CAD build for the part. Positions are in the model's coordinates, mm. Face numbers are marked on the shaded views. Round coordinates to 2 decimals unless told otherwise and drop trailing zeros. Loops run counter-clockwise (first coordinate to the right, second up) from the corner with the lowest first, then second, coordinate; pieces in that order, holes last. Notation, with made-up numbers: (-7, 54.25) - (30, 54.25) arc R28 cw to (30, 78.25) - close; hole circle Ø1 at (78, -1.75). An arc over 180 degrees is marked (long way). Use one line per item in the form item = value.
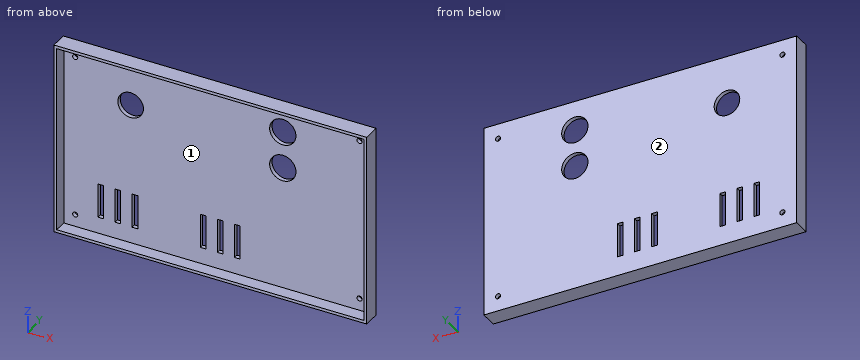
from build123d import *

# Parameters (mm, degrees)
SKETCH_1_W                       = 220
SKETCH_1_H                       = 135
LID_TOP_3MM_DEPTH                = 3
SKETCH_2_W                       = 216
SKETCH_2_H                       = 2
LID_RIM_BACK_DEPTH               = 12
SKETCH_3_W                       = 216
SKETCH_3_H                       = 2
LID_RIM_FRONT_DEPTH              = 12
SKETCH_4_W                       = 2
SKETCH_4_H                       = 135
LID_RIM_LEFT_DEPTH               = 12
SKETCH_5_W                       = 2
SKETCH_5_H                       = 135
LID_RIM_RIGHT_DEPTH              = 12
SKETCH_6_R                       = 1.8
LID_SCREW_CLEARANCE_1_DEPTH      = 16
SKETCH_7_R                       = 1.8
LID_SCREW_CLEARANCE_2_DEPTH      = 16
SKETCH_8_R                       = 1.8
LID_SCREW_CLEARANCE_3_DEPTH      = 16
SKETCH_9_R                       = 1.8
LID_SCREW_CLEARANCE_4_DEPTH      = 16
SKETCH_10_R                      = 9
OV5647_LENS_OPENING_D18_DEPTH    = 4
SKETCH_11_R                      = 9.25
HC_SR04_ACOUSTIC_OPENING_1_DEPTH = 4
SKETCH_12_R                      = 9.25
HC_SR04_ACOUSTIC_OPENING_2_DEPTH = 4
SKETCH_13_W                      = 4
SKETCH_13_H                      = 24
VENT_SLOT_1_DEPTH                = 4
SKETCH_14_W                      = 4
SKETCH_14_H                      = 24
VENT_SLOT_2_DEPTH                = 4
SKETCH_15_W                      = 4
SKETCH_15_H                      = 24
VENT_SLOT_3_DEPTH                = 4
SKETCH_16_W                      = 4
SKETCH_16_H                      = 24
VENT_SLOT_4_DEPTH                = 4
SKETCH_17_W                      = 4
SKETCH_17_H                      = 24
VENT_SLOT_5_DEPTH                = 4
SKETCH_18_W                      = 4
SKETCH_18_H                      = 24
VENT_SLOT_6_DEPTH                = 4


with BuildPart() as part:
    # 草图1 → Lid_Top_3mm (new body)
    with BuildSketch(Plane(origin=(0, 0, 0), x_dir=(1, 0, 0), z_dir=(0, 1, 0))):
        Rectangle(SKETCH_1_W, SKETCH_1_H)
    extrude(amount=-LID_TOP_3MM_DEPTH)

    # 草图2 → Lid_Rim_Back (add)
    with BuildSketch(Plane(origin=(0, 0, 0), x_dir=(1, 0, 0), z_dir=(0, 1, 0))):
        with Locations((0, 66.5)):
            Rectangle(SKETCH_2_W, SKETCH_2_H)
    extrude(amount=-LID_RIM_BACK_DEPTH)

    # 草图3 → Lid_Rim_Front (add)
    with BuildSketch(Plane(origin=(0, 0, 0), x_dir=(1, 0, 0), z_dir=(0, 1, 0))):
        with Locations((0, -66.5)):
            Rectangle(SKETCH_3_W, SKETCH_3_H)
    extrude(amount=-LID_RIM_FRONT_DEPTH)

    # 草图4 → Lid_Rim_Left (add)
    with BuildSketch(Plane(origin=(0, 0, 0), x_dir=(1, 0, 0), z_dir=(0, 1, 0))):
        with Locations((-109, 0)):
            Rectangle(SKETCH_4_W, SKETCH_4_H)
    extrude(amount=-LID_RIM_LEFT_DEPTH)

    # 草图5 → Lid_Rim_Right (add)
    with BuildSketch(Plane(origin=(0, 0, 0), x_dir=(1, 0, 0), z_dir=(0, 1, 0))):
        with Locations((109, 0)):
            Rectangle(SKETCH_5_W, SKETCH_5_H)
    extrude(amount=-LID_RIM_RIGHT_DEPTH)

    # 草图6 → Lid_Screw_Clearance_1 (cut)
    with BuildSketch(Plane(origin=(0, 0, 0), x_dir=(1, 0, 0), z_dir=(0, 1, 0))):
        with Locations(Location((-100, -57, 0), (0, 0, 270))):
            Circle(SKETCH_6_R)
    extrude(amount=-LID_SCREW_CLEARANCE_1_DEPTH, mode=Mode.SUBTRACT)

    # 草图7 → Lid_Screw_Clearance_2 (cut)
    with BuildSketch(Plane(origin=(0, 0, 0), x_dir=(1, 0, 0), z_dir=(0, 1, 0))):
        with Locations(Location((100, -57, 0), (0, 0, 270))):
            Circle(SKETCH_7_R)
    extrude(amount=-LID_SCREW_CLEARANCE_2_DEPTH, mode=Mode.SUBTRACT)

    # 草图8 → Lid_Screw_Clearance_3 (cut)
    with BuildSketch(Plane(origin=(0, 0, 0), x_dir=(1, 0, 0), z_dir=(0, 1, 0))):
        with Locations(Location((-100, 57, 0), (0, 0, 270))):
            Circle(SKETCH_8_R)
    extrude(amount=-LID_SCREW_CLEARANCE_3_DEPTH, mode=Mode.SUBTRACT)

    # 草图9 → Lid_Screw_Clearance_4 (cut)
    with BuildSketch(Plane(origin=(0, 0, 0), x_dir=(1, 0, 0), z_dir=(0, 1, 0))):
        with Locations(Location((100, 57, 0), (0, 0, 270))):
            Circle(SKETCH_9_R)
    extrude(amount=-LID_SCREW_CLEARANCE_4_DEPTH, mode=Mode.SUBTRACT)

    # 草图10 → OV5647_Lens_Opening_D18 (cut)
    with BuildSketch(Plane(origin=(0, 0, 0), x_dir=(1, 0, 0), z_dir=(0, 1, 0))):
        with Locations(Location((-61, -34, 0), (0, 0, 270))):
            Circle(SKETCH_10_R)
    extrude(amount=-OV5647_LENS_OPENING_D18_DEPTH, mode=Mode.SUBTRACT)

    # 草图11 → HC_SR04_Acoustic_Opening_1 (cut)
    with BuildSketch(Plane(origin=(0, 0, 0), x_dir=(1, 0, 0), z_dir=(0, 1, 0))):
        with Locations(Location((46, -47, 0), (0, 0, 270))):
            Circle(SKETCH_11_R)
    extrude(amount=-HC_SR04_ACOUSTIC_OPENING_1_DEPTH, mode=Mode.SUBTRACT)

    # 草图12 → HC_SR04_Acoustic_Opening_2 (cut)
    with BuildSketch(Plane(origin=(0, 0, 0), x_dir=(1, 0, 0), z_dir=(0, 1, 0))):
        with Locations(Location((46, -21, 0), (0, 0, 270))):
            Circle(SKETCH_12_R)
    extrude(amount=-HC_SR04_ACOUSTIC_OPENING_2_DEPTH, mode=Mode.SUBTRACT)

    # 草图13 → Vent_Slot_1 (cut)
    with BuildSketch(Plane(origin=(0, 0, 0), x_dir=(1, 0, 0), z_dir=(0, 1, 0))):
        with Locations((-82, 42)):
            Rectangle(SKETCH_13_W, SKETCH_13_H)
    extrude(amount=-VENT_SLOT_1_DEPTH, mode=Mode.SUBTRACT)

    # 草图14 → Vent_Slot_2 (cut)
    with BuildSketch(Plane(origin=(0, 0, 0), x_dir=(1, 0, 0), z_dir=(0, 1, 0))):
        with Locations((-70, 42)):
            Rectangle(SKETCH_14_W, SKETCH_14_H)
    extrude(amount=-VENT_SLOT_2_DEPTH, mode=Mode.SUBTRACT)

    # 草图15 → Vent_Slot_3 (cut)
    with BuildSketch(Plane(origin=(0, 0, 0), x_dir=(1, 0, 0), z_dir=(0, 1, 0))):
        with Locations((-58, 42)):
            Rectangle(SKETCH_15_W, SKETCH_15_H)
    extrude(amount=-VENT_SLOT_3_DEPTH, mode=Mode.SUBTRACT)

    # 草图16 → Vent_Slot_4 (cut)
    with BuildSketch(Plane(origin=(0, 0, 0), x_dir=(1, 0, 0), z_dir=(0, 1, 0))):
        with Locations((-10, 42)):
            Rectangle(SKETCH_16_W, SKETCH_16_H)
    extrude(amount=-VENT_SLOT_4_DEPTH, mode=Mode.SUBTRACT)

    # 草图17 → Vent_Slot_5 (cut)
    with BuildSketch(Plane(origin=(0, 0, 0), x_dir=(1, 0, 0), z_dir=(0, 1, 0))):
        with Locations((2, 42)):
            Rectangle(SKETCH_17_W, SKETCH_17_H)
    extrude(amount=-VENT_SLOT_5_DEPTH, mode=Mode.SUBTRACT)

    # 草图18 → Vent_Slot_6 (cut)
    with BuildSketch(Plane(origin=(0, 0, 0), x_dir=(1, 0, 0), z_dir=(0, 1, 0))):
        with Locations((14, 42)):
            Rectangle(SKETCH_18_W, SKETCH_18_H)
    extrude(amount=-VENT_SLOT_6_DEPTH, mode=Mode.SUBTRACT)


solid = part.part
1) Slice it at B-B (z = -46). State how many separate pieces and enclosed holes the cut face has, plus the area to 3 significant figures.
Report:
separate_pieces = 7
enclosed_holes = 0
area = 624 mm^2
2) Drill centre lines: probe 1 along Z at (x, y) = (100, -2.3); probe 2 along X at (y, z) = (-1.75, 57); probe 3 along X at (y, z) = (-8.5, -37). Where is each one in solid material? Low to high.
Report:
probe_1 = -67.5 to -58.8, -55.2 to 55.2, 58.8 to 67.5
probe_2 = -110 to -101.8, -98.2 to 98.2, 101.8 to 110
probe_3 = -110 to -108, 108 to 110
3) Flat gauge pins, fed straight in: pin 1 (6 mm diameter, centred on x = 83.5, z = 40, fed in from +Y); pin 2 (21.5 mm diameter, centred on x = 46, z = 21, fed in from -Y). Where does each tip first touch, or does it go through?
Report:
pin_1 = 0
pin_2 = -3
4) Slice it at A-A (z = 21). Write the cut outline in (x, y), plus the area to 4 significant figures.
Report:
outline = (-110, -12) - (-108, -12) - (-108, -3) - (36.75, -3) - (36.75, 0) - (-110, 0) - close; (55.25, -3) - (108, -3) - (108, -12) - (110, -12) - (110, 0) - (55.25, 0) - close
area = 640.5 mm^2
5) Two-plate mould, pull along Z, no slides. Class the marked faces 1 and 2: +Z half, -Z half, draft (parallel to the pull), parting line (faces both ways), or undercut.
Report:
face_1 = undercut
face_2 = draft
6) Slice it at D-D (x = 24.5). Write the cut outline in (y, z), plus the area to 3 significant figures.
Report:
outline = (-12, -67.5) - (0, -67.5) - (0, 67.5) - (-12, 67.5) - (-12, 65.5) - (-3, 65.5) - (-3, -65.5) - (-12, -65.5) - close
area = 441 mm^2
7) Slice it at C-C (y = -6). Write the cut outline in (x, z), plus the area to 3 significant figures.
Report:
outline = (-110, -67.5) - (110, -67.5) - (110, 67.5) - (-110, 67.5) - close; hole (-108, -65.5) - (108, -65.5) - (108, 65.5) - (-108, 65.5) - close
area = 1,400 mm^2
